Source: CAD feature listing. Evaluate the final solid. Frame: model axes, mm. A direction names the side the tool comes from. Coordinates: 2 decimals unless noted, no trailing zeros. Order: outer loops, then holes, each group sorted by start corner. A loop starts at its lowest first (then second) coordinate and runs counter-clockwise, first axis right, second up. Notation, with made-up numbers: (88.25, 31) - (97.25, 31) arc R20 ccw to (97.25, 64) - close; hole circle Ø9 at (-6, 76). An arc over 180 degrees is marked (long way). One line per question, with ' | ' between items. Start each with the question number.
(1) Section D-D (x = 47). Return the cut outline in (y, z).
(2) Access query for faces 1 (the flat face through (12, 90, 3)), 2 (the flat face through (13, 80, 3)), 3 (the flat face through (25, 87, 3)). Directions: +Z, -Z, +X, -X, +Y, -Y. A direction counts if a zero-diameter tool reaches every point of the face in a straight line with its end or side. Return the directions, or none.
(3) Line query: line 1 along Y through (x, z) = (11.5, 0.9); line 2 along X through (y, z) = (61, 3.75); line 3 along Y through (x, z) = (50, 5.35). Output: solid intervals per line, ascending.
(4) Draft query along Y for faces 4 (the flat face through (41.97, 43.27, 2.96)), 5 (the flat face through (0, 44, 3)), 6 (the flat face through (30, 46, 3)), 7 (the flat face through (30, 0, 3)). Return one class per face: +Y half, -Y half, draft (parallel to the pull), parting line (faces both ways), or undercut.
(5) Contact query for flat-ended pins moving along their axis: P1, Ø3, axis at y = 30, z = 2.5, coming from the +X side (3 decimals); P2, Ø1, axis at y = 22, z = 3, coming from the +X side. Output: stop coordinate, or through.
(6) Section A-A (x = 13.5). Return the cut outline in (y, z), then the cut area to 3 significant figures.
(7) Section B-B (z = 4.6). Return the cut outline in (x, y).
(8) Section C-C (y = 63). Return the cut outline in (x, z).
from build123d import *

# Parameters (mm, degrees)
BOSS_EXTRU_1_DEPTH = 6


with BuildPart() as part:
    # Esquisse1 → Boss.-Extru.1 (new body)
    with BuildSketch(Plane.XY):
        with BuildLine():
            Line((0, 1), (0, 89))
            ThreePointArc((0, 89), (0.292893219, 89.707106781), (1, 90))
            Line((1, 90), (24, 90))
            ThreePointArc((24, 90), (24.707106781, 89.707106781), (25, 89))
            Line((25, 89), (25, 84))
            Line((25, 84), (59.423076923, 1.384615385))
            ThreePointArc((59.423076923, 1.384615385), (59.332050294, 0.445299804), (58.5, 0))
            Line((58.5, 0), (1, 0))
            ThreePointArc((1, 0), (0.292893219, 0.292893219), (0, 1))
        make_face()
        with BuildLine():
            Line((10, 11), (10, 79))
            ThreePointArc((10, 79), (10.292893219, 79.707106781), (11, 80))
            Line((11, 80), (15.166666667, 80))
            ThreePointArc((15.166666667, 80), (15.721366863, 79.832050294), (16.08974359, 79.384615385))
            Line((16.08974359, 79.384615385), (44.423076923, 11.384615385))
            ThreePointArc((44.423076923, 11.384615385), (44.332050294, 10.445299804), (43.5, 10))
            Line((43.5, 10), (11, 10))
            ThreePointArc((11, 10), (10.292893219, 10.292893219), (10, 11))
        make_face(mode=Mode.SUBTRACT)
    extrude(amount=BOSS_EXTRU_1_DEPTH)


solid = part.part
Response values:
1) outline: (0, 0) - (31.2, 0) - (31.2, 6) - (0, 6) - close
2) face 1: +Z, -Z, +X, -X, +Y | face 2: +Z, -Z | face 3: +Z, -Z, +X, +Y
3) line 1: y = 0 to 10, 80 to 90 | line 2: x = 0 to 10, 23.75 to 34.58 | line 3: y = 0 to 24
4) face 4: +Y half | face 5: draft | face 6: undercut | face 7: -Y half
5) P1: stops at x = 48.125 | P2: stops at x = 51.04
6) outline: (0, 0) - (10, 0) - (10, 6) - (0, 6) - close; (80, 0) - (90, 0) - (90, 6) - (80, 6) - close | area: 120 mm²
7) outline: (0, 1) arc R1 ccw to (1, 0) - (58.5, 0) arc R1 ccw to (59.42, 1.38) - (25, 84) - (25, 89) arc R1 ccw to (24, 90) - (1, 90) arc R1 ccw to (0, 89) - close; hole (10, 11) arc R1 ccw to (11, 10) - (43.5, 10) arc R1 ccw to (44.42, 11.38) - (16.09, 79.38) arc R1 ccw to (15.17, 80) - (11, 80) arc R1 ccw to (10, 79) - close
8) outline: (0, 0) - (10, 0) - (10, 6) - (0, 6) - close; (22.92, 0) - (33.75, 0) - (33.75, 6) - (22.92, 6) - close
